```python
from build123d import *

# Parameters (mm, degrees)
SKETCH_1_R                   = 6
EXTRUDE_1_DEPTH              = 47
EXTRUDE_2_DEPTH              = 1.8
EXTRUDE_2_DEPTH_BACK         = 1.8
SKETCH_2_W                   = 20
SKETCH_2_H                   = 4
HOLE_WIZARD_M2_2_D           = 2.4
HOLE_WIZARD_M2_2_DEPTH       = 5
HOLE_WIZARD_M2_2_CSINK_D     = 4.55
HOLE_WIZARD_M2_2_CSINK_ANGLE = 90
HOLE_WIZARD_M2_2_TIP         = 0.721032743
HOLE_WIZARD_M2_3_D           = 2.4
HOLE_WIZARD_M2_3_DEPTH       = 5
HOLE_WIZARD_M2_3_CSINK_D     = 4.55
HOLE_WIZARD_M2_3_CSINK_ANGLE = 90
HOLE_WIZARD_M2_3_TIP         = 0.721032743


with BuildPart() as part:
    # 스케치1 → 보스-돌출1 (new body)
    with BuildSketch(Plane.XY):
        Circle(SKETCH_1_R)
    extrude(amount=EXTRUDE_1_DEPTH)

    # 스케치2 → 보스-돌출2 (add, two sides: drawn at the far end of the back side and taken through both)
    with BuildSketch(Plane(origin=(0, 6, 0), x_dir=(0, 0, -1), z_dir=(0, 1, 0)).offset(-EXTRUDE_2_DEPTH_BACK)):
        with Locations((-34, 0)):
            Rectangle(SKETCH_2_W, SKETCH_2_H)
    extrude(amount=EXTRUDE_2_DEPTH + EXTRUDE_2_DEPTH_BACK)

    # M2 여유 구멍2
    with Locations(Plane.XY.offset(47)):
        with Locations((0, 0)):
            CounterSinkHole(HOLE_WIZARD_M2_2_D / 2, HOLE_WIZARD_M2_2_CSINK_D / 2, depth=HOLE_WIZARD_M2_2_DEPTH, counter_sink_angle=HOLE_WIZARD_M2_2_CSINK_ANGLE)
            with Locations((0, 0, -(HOLE_WIZARD_M2_2_DEPTH + HOLE_WIZARD_M2_2_TIP / 2))):  # 118° drill point
                Cone(0, HOLE_WIZARD_M2_2_D / 2, HOLE_WIZARD_M2_2_TIP, mode=Mode.SUBTRACT)

    # M2 여유 구멍3
    with Locations(Plane(origin=(0, 0, 0), x_dir=(-1, 0, 0), z_dir=(0, 0, -1))):
        with Locations((0, 0)):
            CounterSinkHole(HOLE_WIZARD_M2_3_D / 2, HOLE_WIZARD_M2_3_CSINK_D / 2, depth=HOLE_WIZARD_M2_3_DEPTH, counter_sink_angle=HOLE_WIZARD_M2_3_CSINK_ANGLE)
            with Locations((0, 0, -(HOLE_WIZARD_M2_3_DEPTH + HOLE_WIZARD_M2_3_TIP / 2))):  # 118° drill point
                Cone(0, HOLE_WIZARD_M2_3_D / 2, HOLE_WIZARD_M2_3_TIP, mode=Mode.SUBTRACT)


solid = part.part
```
Geometry check sheet. Reference: the model listing, model coordinates, mm. A direction names the side the tool comes from. Coordinates: 2 decimals unless noted, no trailing zeros. Loops run counter-clockwise (first coordinate to the right, second up) from the corner with the lowest first, then second, coordinate; pieces in that order, holes last. Notation, with made-up numbers: (-10, -39.75) -> (41, -39.75) arc R19 ccw to (41, -24.75) -> close; hole circle Ø1 at (38.25, 59). An arc over 180 degrees is marked (long way). Put each result on its own line as item: value.
1) Thickness scan on line 1 (Y direction, x = 0, z = 43.2); line 2 (Y direction, x = 0, z = 44.75); line 3 (X direction, y = 5.75, z = 41.5). Record the ranges inside material, lowest first.
Result set:
line 1: y = -6 to -1.2, 1.2 to 7.8
line 2: y = -6 to -1.2, 1.2 to 6
line 3: x = -2 to 2
2) Cross-section at A-A on z = 30. Record the boundary of the cut face in (x, y).
Result set:
outline: (-2, 5.66) arc R6 ccw (long way) to (2, 5.66) -> (2, 7.8) -> (-2, 7.8) -> close
3) Cross-section at C-C on z = 11. Record the boundary of the cut face in (x, y).
Result set:
outline: circle Ø12 at (0, 0)
4) Gauge pin test, flat ends, axial feed: pin 1 Ø3 at (x, y) = (0, 0) entering from -Z (3 decimals); pin 2 Ø1.5 at (y, z) = (1, 16.5) entering from -X; pin 3 Ø0.6 at (y, z) = (7, 30.5) entering from +X. Record the tip position at first contact, or that the pin passes through.
Result set:
pin 1: stops at z = 0.775
pin 2: stops at x = -5.99
pin 3: stops at x = 2
5) Cross-section at B-B on y = 4.5. Record the boundary of the cut face in (x, z), plus the area to 3 significant figures.
Result set:
outline: (-3.97, 0) -> (3.97, 0) -> (3.97, 47) -> (-3.97, 47) -> close
area: 373 mm^2
6) Release check for a two-part mould opening along Y. For faces 1 (the flat face through (-2, 7, 34)), 2 (the cylindrical face through (-1.301, -5.857, 23.171)), 3 (the conical face through (0, -0.2, 41.4)) record: released by +Y, released by -Y, zero draft, split by the parting line, or undercut.
Result set:
face 1: zero draft
face 2: split by the parting line
face 3: undercut
7) Tool access check on faces 4 (the cylindrical face through (-0.65, 1.01, 43.94)), 5 (the flat face through (2, 7, 34)), 6 (the cylindrical face through (0.65, 1.01, 3.06)), 7 (the flat face through (0, 7.8, 34)), 8 (the flat face through (3, 0, 0)). Record the directions out of +Z, -Z, +X, -X, +Y, -Y that give a thin tool (end or side, any length) a straight path to the whole face; none if there is none.
Result set:
face 4: +Z
face 5: +Z, -Z, +X, +Y
face 6: -Z
face 7: +Z, -Z, +X, -X, +Y
face 8: -Z, +X, -X, +Y, -Y
